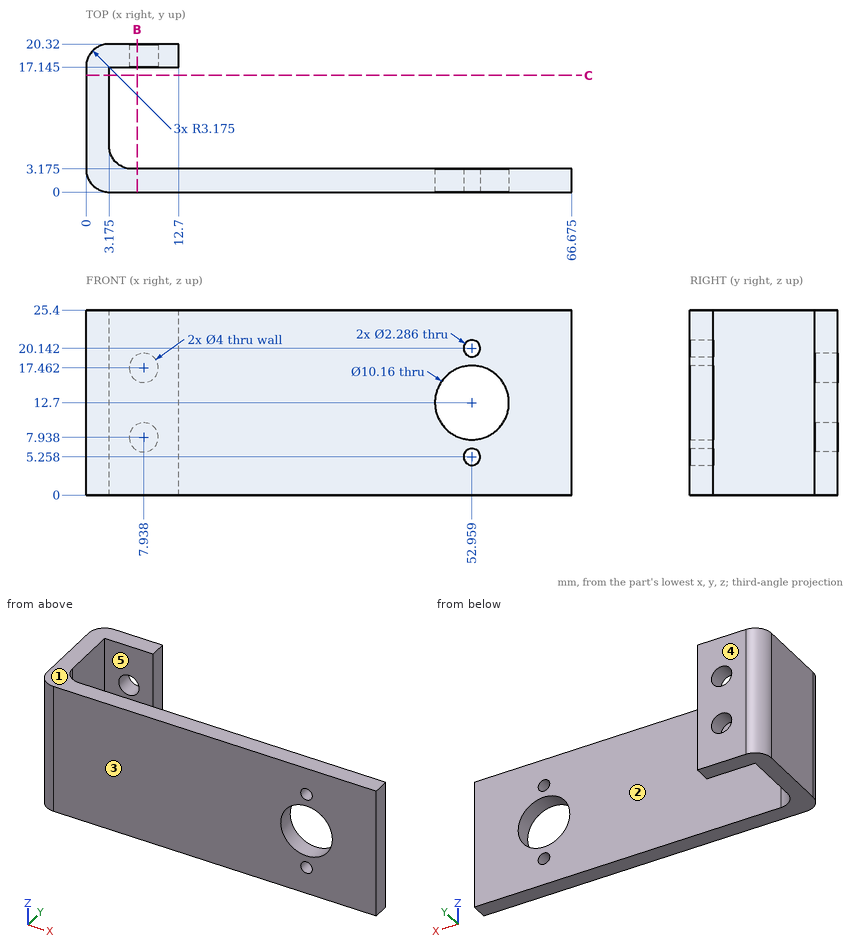
Input: dimensioned drawing with shaded views. Units: mm. Origin: part minimum x, y, z. A direction names the side the tool comes from. Give positions to 0.01 mm unless a question says otherwise; leave off trailing zeros. Write each loop counter-clockwise with the first axis right and the second up, starting at its lowest first coordinate (ties: lowest second). Pieces come first, ordered by that corner, then holes.
Q1. Material intervals for probe 1 along Y at (x, z) = (8, 4) (1 decimal); probe 2 along X at (y, z) = (2, 13.75) (1 decimal); probe 3 along Y at (x, z) = (35, 1.5) (1 decimal), sorted ascending.
Q2. Section B-B, the plane x = 7. Output: boundary loops of the cut face in (y, z) (1 decimal).
Q3. Pull-direction query (Y, two-part tool) for the marked faces 3, 4 and 5; classes: pulls with the +Y half, pulls with the -Y half, needs draft (parallel to the pull), parting line crosses it, or undercut.
Q4. First-contact query: P1, Ø12, axis at y = 9.5, z = 18.5, coming from the +X side; P2, Ø1.6, axis at y = 18, z = 14.5, coming from the +X side; P3, Ø1, axis at x = 43, z = 20.5, coming from the -Y side; P4, Ø1.5, axis at x = 34, z = 10, coming from the +Y side (1 decimal). Flat tips, straight axial feed; report the tip coordinate or a pass-through.
Q5. Set-up query: the marked faces 1 and 2. Return all of +Z, -Z, +X, -X, +Y, -Y with unobstructed straight access to the full face (end or side cutting, diameter ignored); none if empty.
Q6. Section C-C, the plane y = 16. Output: boundary loops of the cut face in (x, z) (1 decimal).
Filled in:
1. probe 1: y = 0 to 3.2, 17.1 to 20.3
1. probe 2: x = 0.2 to 48, 57.9 to 66.7
1. probe 3: y = 0 to 3.2
2. outline: (0, 0) - (3.2, 0) - (3.2, 25.4) - (0, 25.4) - close; (17.1, 0) - (20.3, 0) - (20.3, 6.2) - (17.1, 6.2) - close; (17.1, 9.7) - (20.3, 9.7) - (20.3, 15.7) - (17.1, 15.7) - close; (17.1, 19.2) - (20.3, 19.2) - (20.3, 25.4) - (17.1, 25.4) - close
3. face 3: pulls with the -Y half
3. face 4: pulls with the +Y half
3. face 5: undercut
4. P1: stops at x = 4.95
4. P2: stops at x = 12.7
4. P3: stops at y = 0
4. P4: stops at y = 3.2
5. face 1: +Z, +X, -X, +Y, -Y
5. face 2: +Z, -Z, +X
6. outline: (0, 0) - (3.2, 0) - (3.2, 25.4) - (0, 25.4) - close
